from build123d import *

# Parameters (mm, degrees)
F0_R      = 8.5
F1_DEPTH  = 20
F2_R      = 10
F3_DEPTH  = 4.83
F4_R      = 15
F5_DEPTH  = 35.4
F6_R      = 16
F7_DEPTH  = 64.6
F8_R      = 15
F9_DEPTH  = 35.4
F10_R     = 10
F11_DEPTH = 4.33
F12_R     = 9
F13_DEPTH = 20
F15_W     = 20
F15_H     = 4
F16_DEPTH = 5


with BuildPart() as f1:
    # F0 (on Right) → F1 (new body)
    with BuildSketch(Plane.YZ):
        Circle(F0_R)
    extrude(amount=F1_DEPTH)

    # F2 (on face) → F3 (join)
    with BuildSketch(Plane.YZ.offset(20)):
        Circle(F2_R)
    extrude(amount=F3_DEPTH)

    # F4 (on face) → F5 (join)
    with BuildSketch(Plane.YZ.offset(24.83)):
        Circle(F4_R)
    extrude(amount=F5_DEPTH)

    # F6 (on face) → F7 (join)
    with BuildSketch(Plane.YZ.offset(60.23)):
        Circle(F6_R)
    extrude(amount=F7_DEPTH)

    # F8 (on face) → F9 (join)
    with BuildSketch(Plane.YZ.offset(124.83)):
        Circle(F8_R)
    extrude(amount=F9_DEPTH)

    # F10 (on face) → F11 (join)
    with BuildSketch(Plane.YZ.offset(160.23)):
        Circle(F10_R)
    extrude(amount=F11_DEPTH)

    # F12 (on face) → F13 (join)
    with BuildSketch(Plane.YZ.offset(164.56)):
        Circle(F12_R)
    extrude(amount=F13_DEPTH)

    # F15 (on offset) → F16 (cut)
    with BuildSketch(Plane.XY.offset(15)):
        with Locations((42.53, 2)):
            Rectangle(F15_W, F15_H)
        with Locations((42.53, -2)):
            Rectangle(F15_W, F15_H)
        with Locations((142.53, 2)):
            Rectangle(F15_W, F15_H)
        with Locations((142.53, -2)):
            Rectangle(F15_W, F15_H)
    extrude(amount=-F16_DEPTH, mode=Mode.SUBTRACT)


solid = f1.part
Work out the finished part from the listing and answer in its coordinate system (mm). A direction names the side the tool comes from. Coordinates: 2 decimals unless noted, no trailing zeros. Loops run counter-clockwise (first coordinate to the right, second up) from the corner with the lowest first, then second, coordinate; pieces in that order, holes last. Notation, with made-up numbers: M 83.5,26.25 L 110.5,26.25 A16 ccw 110.5,48.25 Z; hole C -31,18 d3. An arc over 180 degrees is marked long. Answer in a Markdown table with one row per item. Add a question column.
1. Find section B-B, the plane x = 55. Write down the section's boundary in (y, z).
2. Consider L1, parallel to X at y = -3, z = 8; L2, parallel to X at y = -10, z = -6; L3, parallel to Y at x = 141, z = -1. Determine where each line is inside the solid, lowest interval first.
3. Find section A-A, the plane z = 0. Write down the section's boundary in (x, y), then the cut area to 3 significant figures.
4. A tool of negligible diameter and unlimited length cuts with its end or side. For faces 1 (the cylindrical face through (142.282, -3.252, -14.643)), 2 (the cylindrical face through (22.38, -2.17, -9.76)), 3 (the flat face through (42, 4, 12)), from which of +Z, -Z, +X, -X, +Y, -Y can it reach the whole face along a straight path? Write none if from no direction.
5. Flat-ended cylindrical pins translate along their axes: P1, Ø2, axis at y = 10, z = 4, coming from the -X side; P2, Ø9, axis at x = 146, y = 0.5, coming from the +Z side; P3, Ø1.3, axis at x = 47, z = 13, coming from the +Y side. Find the tip coordinate at first contact, or state that the pin passes through.
6. Find section C-C, the plane y = -6.5. Write down the section's boundary in (x, z).
7. The mould has two halves that part along Y. Classify faces 4 (the cylindrical face through (42.282, -3.252, -14.643)), 5 (the flat face through (0, 0, 0)), 6 (the flat face through (52.53, 0, 13)): pulls with the +Y half, pulls with the -Y half, needs draft (parallel to the pull), parting line crosses it, or undercut.
Reported:
| question | item | result |
|---|---|---|
| 1 | outline | C 0,0 d30 |
| 2 | L1 | x = 20 to 184.56 |
| 2 | L2 | x = 24.83 to 160.23 |
| 2 | L3 | y = -14.97 to 14.97 |
| 3 | outline | M 0,-8.5 L 20,-8.5 L 20,-10 L 24.83,-10 L 24.83,-15 L 60.23,-15 L 60.23,-16 L 124.83,-16 L 124.83,-15 L 160.23,-15 L 160.23,-10 L 164.56,-10 L 164.56,-9 L 184.56,-9 L 184.56,9 L 164.56,9 L 164.56,10 L 160.23,10 L 160.23,15 L 124.83,15 L 124.83,16 L 60.23,16 L 60.23,15 L 24.83,15 L 24.83,10 L 20,10 L 20,8.5 L 0,8.5 Z |
| 3 | area | 5,070 mm^2 |
| 4 | face 1 | +X |
| 4 | face 2 | -X |
| 4 | face 3 | +Z |
| 5 | P1 | stops at x = 20 |
| 5 | P2 | stops at z = 14.46 |
| 5 | P3 | stops at y = 8.51 |
| 6 | outline | M 0,-5.48 L 20,-5.48 L 20,-7.6 L 24.83,-7.6 L 24.83,-13.52 L 60.23,-13.52 L 60.23,-14.62 L 124.83,-14.62 L 124.83,-13.52 L 160.23,-13.52 L 160.23,-7.6 L 164.56,-7.6 L 164.56,-6.22 L 184.56,-6.22 L 184.56,6.22 L 164.56,6.22 L 164.56,7.6 L 160.23,7.6 L 160.23,13.52 L 124.83,13.52 L 124.83,14.62 L 60.23,14.62 L 60.23,13.52 L 24.83,13.52 L 24.83,7.6 L 20,7.6 L 20,5.48 L 0,5.48 Z |
| 7 | face 4 | parting line crosses it |
| 7 | face 5 | needs draft |
| 7 | face 6 | undercut |
